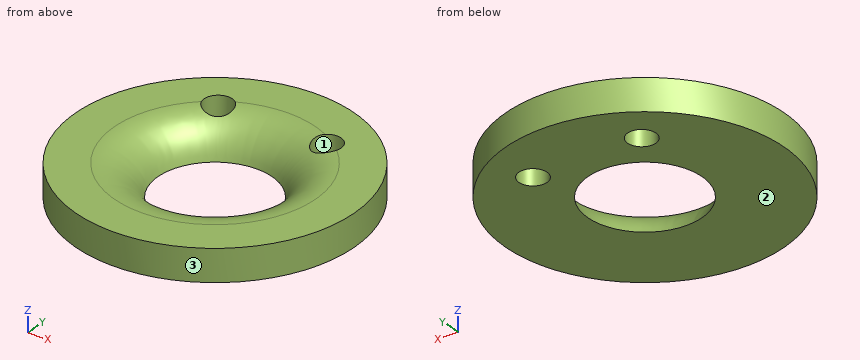
from build123d import *

# Parameters (mm, degrees)
SKETCH1_R                        = 30.5
BOSS_EXTRUDE1_DEPTH              = 7
SKETCH2_R                        = 3.1
F_2X_6_2_MM_AND_25_MM_THRU_DEPTH = 44.697826033
F_10MM_FILET_R                   = 10


with BuildPart() as part:
    # Sketch1 → Boss-Extrude1 (new body)
    with BuildSketch(Plane(origin=(0, 0, 0), x_dir=(0, 1, 0), z_dir=(0, 0, 1))):
        with Locations(Location((0, 0, 0), (0, 0, 270))):
            Circle(SKETCH1_R)
    extrude(amount=BOSS_EXTRUDE1_DEPTH)

    # Sketch2 → 2x 6.2 mm and 25 mm thru (cut, through all)
    with BuildSketch(Plane.XY.offset(7)):
        with BuildLine():
            ThreePointArc((12.5, 0), (8.838834765, 8.838834765), (0, 12.5))
            Line((0, 12.5), (0, -12.5))
            ThreePointArc((0, -12.5), (8.838834765, -8.838834765), (12.5, 0))
        make_face()
        with BuildLine():
            Line((0, -12.5), (0, 12.5))
            ThreePointArc((0, 12.5), (-12.5, 0), (0, -12.5))
        make_face()
        with Locations((-11.907432919, 17.394401462)):
            Circle(SKETCH2_R)
        with Locations((11.907432919, 17.394401462)):
            Circle(SKETCH2_R)
    extrude(amount=-F_2X_6_2_MM_AND_25_MM_THRU_DEPTH, mode=Mode.SUBTRACT)

    # 10mm filet
    # the kernel refuses this fillet: 10 mm, written as the material it takes off along each edge
    with BuildSketch(Plane(origin=(0, 0, 7), x_dir=(0, -1, 0), z_dir=(1, 0, 0))) as f_10mm_filet_piece_1:
        with BuildLine():
            CenterArc((22.039392014, 10), F_10MM_FILET_R, 197.457603124, 72.542396876)
            Line((12.5, 7), (12.30921216, 6.94))
            ThreePointArc((12.30921216, 6.94), (12.3, 3.5), (12.3, 0))
            Line((12.3, 0), (12.5, -0.2))
            Line((12.5, -0.2), (22.039392014, -0.2))
            Line((22.039392014, -0.2), (22.039392014, 0))
        make_face()
    revolve(axis=Axis((0, 0, 7), (0, 0, -1)), mode=Mode.SUBTRACT)


solid = part.part
Read the model definition and answer for the solid it produces. Units are mm, in the model's axes. Face numbers are marked on the shaded views. Give positions to 0.01 mm unless a question says otherwise; leave off trailing zeros. Loops run counter-clockwise (first coordinate to the right, second up) from the corner with the lowest first, then second, coordinate; pieces in that order, holes last. Notation, with made-up numbers: (-21, -40) - (33, -40) arc R22 cw to (33, -13) - close; hole circle Ø6 at (80, 19.5). An arc over 180 degrees is marked (long way). Answer as CSV lines item,"result". Start each with the question number.
1) Find section C-C (z = 2.25). Write down the section's boundary in (x, y).
2) Each of these flat-tipped pins is pushed along its axis until it touches: pin 1 Ø3 at (y, z) = (11.5, 6) entering from -X; pin 2 Ø1 at (x, z) = (15.5, 6) entering from -Y; pin 3 Ø2 at (y, z) = (16.5, 5) entering from +X. Where does it stop, or does it pass through?
3) Straight lines are drawn through the part: L1, parallel to Y at x = -12.5, z = 5; L2, parallel to X at y = -1, z = 0.5; L3, parallel to X at y = 2.5, z = 5.75. For each, find the intervals that lie inside material, in ascending order. Write a range as from..to.
4) Determine the mould class of the marked faces 1, 2 and 3 for opening direction Y: released by +Y, released by -Y, zero draft, split by the parting line, or undercut.
5) Find section A-A (x = 0). Write down the section's boundary in (y, z), then the cut area to 3 significant figures.
Findings below:
1,outline,"circle Ø61 at (0, 0); hole circle Ø6.2 at (-11.91, 17.39); hole circle Ø27.06 at (0, 0); hole circle Ø6.2 at (11.91, 17.39)"
2,pin 1,"x = -28.81"
2,pin 2,"y = -26.56"
2,pin 3,"x = 26.27"
3,L1,"-27.82..-10.05, 10.05..14.35, 20.44..27.82"
3,L2,"-30.48..-12.63, 12.63..30.48"
3,L3,"-30.4..-17.02, 17.02..30.4"
4,face 1,"undercut"
4,face 2,"zero draft"
4,face 3,"split by the parting line"
5,outline,"(-30.5, 0) - (-12.5, 0) arc R10 ccw to (-22.04, 7) - (-30.5, 7) - close; (12.5, 0) - (30.5, 0) - (30.5, 7) - (22.04, 7) arc R10 ccw to start"
5,area,"216 mm^2"
